The model under review builds one solid part; all positions refer to its coordinate system, in mm. A direction names the side the tool comes from. Coordinates: 2 decimals unless noted, no trailing zeros. Write each loop counter-clockwise with the first axis right and the second up, starting at its lowest first coordinate (ties: lowest second). Pieces come first, ordered by that corner, then holes. Notation, with made-up numbers: (66, -22.5) - (91, -22.5) arc R37 cw to (91, 16.5) - close; hole circle Ø9 at (-17.75, 47). An arc over 180 degrees is marked (long way). Use one line per item in the form item = value. Start each with the question number.
```python
from build123d import *

# Parameters (mm, degrees)
PAD004_DEPTH       = 23
PAD005_DEPTH       = 44
SKETCH007_W        = 43
SKETCH007_H        = 35
POCKET001_DEPTH    = 53
PAD006_DEPTH       = 25
SKETCH009_R        = 1.5
POCKET002_DEPTH    = 44.001
SKETCH012_R        = 3
POCKET004_DEPTH    = 10
POLARPATTERN_COUNT = 4
CHAMFER_SIZE       = 5
POCKET_DEPTH       = 5
PAD_DEPTH          = 44
SKETCH014_R        = 1.5
POCKET005_DEPTH    = 57.001
PAD007_DEPTH       = 15
SKETCH016_R        = 1.5
POCKET006_DEPTH    = 20
SKETCH017_R        = 1.5
POCKET007_DEPTH    = 20
SKETCH018_W        = 9
SKETCH018_H        = 10
POCKET008_DEPTH    = 15
POCKET009_DEPTH    = 15
SKETCH020_R        = 1.5
POCKET010_DEPTH    = 5


with BuildPart() as part:
    # Sketch005 → Pad004 (new body)
    with BuildSketch(Plane.XY):
        Polygon((32, -42), (32, 32), (-32, 32), (-32, -42), (-20, -42), (-20, 20), (20, 20), (20, -42), align=None)
    extrude(amount=-PAD004_DEPTH)

    # Sketch006 (on Face10 of Pad004) → Pad005 (join)
    with BuildSketch(Plane(origin=(0, 0, -23), x_dir=(1, 0, 0), z_dir=(0, 0, -1))):
        with BuildLine():
            Line((-25, 57), (-25, -1))
            Line((-25, -1), (25, -1))
            Line((25, -1), (25, 57))
            Line((25, 57), (12, 57))
            Line((12, 28.000302), (12, 57))
            ThreePointArc((-12, 27.999702), (0.0003, 16), (12, 28.000302))
            Line((-12, 27.999702), (-12, 57))
            Line((-12, 57), (-25, 57))
        make_face()
    extrude(amount=PAD005_DEPTH)

    # Sketch007 (on Face16 of Pad005) → Pocket001 (cut)
    with BuildSketch(Plane.XZ.offset(57)):
        with Locations((0, -45.217157)):
            Rectangle(SKETCH007_W, SKETCH007_H)
    extrude(amount=-POCKET001_DEPTH, mode=Mode.SUBTRACT)

    # Sketch008 (on Face9 of Pocket001) → Pad006 (join)
    with BuildSketch(Plane.XZ.offset(42)):
        Polygon((-32, -23), (-25, -23), (-25, -42.561909), align=None)
        Polygon((32, -23), (25, -23), (25, -42.561909), align=None)
    extrude(amount=-PAD006_DEPTH)

    # Sketch009 (on Face7 of Pad006) → Pocket002 (cut, through all)
    with BuildSketch(Plane.XY.offset(-23)):
        with Locations((-15.5, -12.5)):
            Circle(SKETCH009_R)
        with Locations((-15.5, -43.5)):
            Circle(SKETCH009_R)
        with Locations((15.5, -43.5)):
            Circle(SKETCH009_R)
        with Locations((15.5, -12.5)):
            Circle(SKETCH009_R)
    extrude(amount=-POCKET002_DEPTH, mode=Mode.SUBTRACT)

    # Sketch012 (on Face4 of Pocket002) → Pocket004 (cut)
    with BuildSketch(Plane.XY):
        with Locations((-25, 25)):
            Circle(SKETCH012_R)
    pocket004 = extrude(amount=-POCKET004_DEPTH, mode=Mode.SUBTRACT)

    # PolarPattern: Pocket004 ×4 about axis
    polarpattern_axis = Axis((0, 0, 0), (0, 0, 1))
    for i in range(1, POLARPATTERN_COUNT):
        add(pocket004.rotate(polarpattern_axis, i * 360 / POLARPATTERN_COUNT), mode=Mode.SUBTRACT)

    # Chamfer
    chamfer_edges = [part.edges().sort_by_distance(p)[0] for p in [
        (-32, 32, -11.5),
        (32, 32, -11.5),
        (-25, 1, -45),
        (25, 1, -45),
        (20, 20, -11.5),
        (-20, 20, -11.5),
    ]]
    chamfer(chamfer_edges, length=CHAMFER_SIZE)

    # Sketch013 (on Face37 of Chamfer) → Pocket (cut)
    with BuildSketch(Plane(origin=(0, 1, 0), x_dir=(-1, 0, 0), z_dir=(0, 1, 0))):
        with BuildLine():
            Line((-12, -62.717157), (12, -62.717157))
            Line((12, -62.717157), (12, -49.356773))
            ThreePointArc((12, -49.356773), (0, -37.356773), (-12, -49.356773))
            Line((-12, -49.356773), (-12, -62.717157))
        make_face()
    extrude(amount=-POCKET_DEPTH, mode=Mode.SUBTRACT)

    # Sketch (on Face5 of Pocket) → Pad (join)
    with BuildSketch(Plane(origin=(0, 0, -23), x_dir=(1, 0, 0), z_dir=(0, 0, -1))):
        Polygon((-32, 17), (-25, 17), (-25, 7), (-20, 2), (-20, -15), (-15, -20), (15, -20), (20, -15), (20, 2), (25, 7), (25, 17), (32, 17), (32, -27), (27, -32), (-27, -32), (-32, -27), align=None)
    extrude(amount=PAD_DEPTH)

    # Sketch014 (on Face13 of Pad) → Pocket005 (cut, through all)
    with BuildSketch(Plane(origin=(-25, 0, 0), x_dir=(0, -1, 0), z_dir=(-1, 0, 0))):
        with Locations((49.5, -33)):
            Circle(SKETCH014_R)
        with Locations((49.5, -56)):
            Circle(SKETCH014_R)
    extrude(amount=-POCKET005_DEPTH, mode=Mode.SUBTRACT)

    # Sketch015 (on Face26 of Pocket005) → Pad007 (join)
    with BuildSketch(Plane(origin=(-25, 0, 0), x_dir=(0, -1, 0), z_dir=(-1, 0, 0))):
        Polygon((22, -67), (42, -67), (42, -47), align=None)
    pad007 = extrude(amount=PAD007_DEPTH)

    # Sketch016 (on Face53 of Pad007) → Pocket006 (cut)
    with BuildSketch(Plane.XZ.offset(42)):
        with Locations((-32.5, -57)):
            Circle(SKETCH016_R)
    pocket006 = extrude(amount=-POCKET006_DEPTH, mode=Mode.SUBTRACT)

    # Sketch017 (on Face20 of Pocket006) → Pocket007 (cut)
    with BuildSketch(Plane(origin=(0, 0, -67), x_dir=(1, 0, 0), z_dir=(0, 0, -1))):
        with Locations((-32.5, 32)):
            Circle(SKETCH017_R)
    pocket007 = extrude(amount=-POCKET007_DEPTH, mode=Mode.SUBTRACT)

    # Sketch018 (on Face20 of Pocket007) → Pocket008 (cut)
    with BuildSketch(Plane(origin=(0, 0, -62), x_dir=(1, 0, 0), z_dir=(0, 0, -1))):
        with Locations((-32.5, 32)):
            Rectangle(SKETCH018_W, SKETCH018_H)
    pocket008 = extrude(amount=-POCKET008_DEPTH, mode=Mode.SUBTRACT)

    # Mirrored: Pad007, Pocket006, Pocket007, Pocket008 across YZ
    add(pad007.mirror(Plane.YZ))
    add(pocket006.mirror(Plane.YZ), mode=Mode.SUBTRACT)
    add(pocket007.mirror(Plane.YZ), mode=Mode.SUBTRACT)
    add(pocket008.mirror(Plane.YZ), mode=Mode.SUBTRACT)

    # Sketch019 (on Face5 of Mirrored) → Pocket009 (cut)
    with BuildSketch(Plane(origin=(0, 32, 0), x_dir=(-1, 0, 0), z_dir=(0, 1, 0))):
        with BuildLine():
            Line((-8, -63), (8, -63))
            Line((8, -63), (8, -50.411114))
            ThreePointArc((8, -50.411114), (0, -42.484996), (-8, -50.411114))
            Line((-8, -50.411114), (-8, -63))
        make_face()
    extrude(amount=-POCKET009_DEPTH, mode=Mode.SUBTRACT)

    # Sketch020 (on Face23 of Pocket009) → Pocket010 (cut)
    with BuildSketch(Plane.XY.offset(-63)):
        with Locations((0, 27.5)):
            Circle(SKETCH020_R)
    extrude(amount=-POCKET010_DEPTH, mode=Mode.SUBTRACT)


solid = part.part
```
1. For P1, Ø5, axis at y = 1.5, z = -36.5, coming from the +X side; P2, Ø4, axis at y = -45.5, z = -25.5, coming from the -X side; P3, Ø10, axis at x = 9.5, y = -29.5, coming from the +Z side, all flat-tipped, find the tip position at first contact; note any pin that passes through.
2. Take a section at D-D (x = 4.5). State the section outline as (y, z) points.
3. Take a section at C-C (z = -5). State the section outline as (x, y) points.
4. For L1, parallel to X at y = 5, z = -40; L2, parallel to Z at x = -3, y = -7.5; L3, parallel to Y at x = 15.5, z = -24.3, list the stretches that pass through material, from the lowest coordinate up.
5. For faces 4 (the flat face through (-30.7, -42, -57.1)), 5 (the flat face through (-34, -33, -62)), 6 (the flat face through (0, 20, -26)), 7 (the flat face through (-20, -8, -18)), 8 (the flat face through (-12, -42, -25)), list the 3-axis set-ups (+Z, -Z, +X, -X, +Y, -Y) from which the entire face can be reached by the end or side of a thin tool; tool diameter is ignored.
6. The part is to be moulded in two halves that separate along X. For faces 1 (the flat face through (30, 29, -33)), 2 (the flat face through (12, -42, -25)), 3 (the cylindrical face through (23.2, -48.3, -33.9)), say which applies: released by +X, released by -X, zero draft, split by the parting line, or undercut.
7. Take a section at B-B (z = -33). Count the separate pieces of the cut face and the enclosed holes in it, plus the area to 3 significant figures.
8. Take a section at A-A (y = -12.5). State the section outline as (x, z) points.
Returned:
q1.P1 = 32
q1.P2 = -25
q1.P3 = -23
q2.outline = (-16.88, -67) - (1, -67) - (1, -62.72) - (-16.88, -62.72) - close; (-16.88, -27.72) - (-4, -27.72) - (-4, -38.23) - (1, -38.23) - (1, -23) - (-16.88, -23) - close; (20, -67) - (32, -67) - (32, -63) - (20, -63) - close; (20, -43.87) - (32, -43.87) - (32, 0) - (20, 0) - close
q3.outline = (-32, -42) - (-20, -42) - (-20, 15) - (-15, 20) - (15, 20) - (20, 15) - (20, -42) - (32, -42) - (32, 27) - (27, 32) - (-27, 32) - (-32, 27) - close; hole circle Ø6 at (-25, -25); hole circle Ø6 at (-25, 25); hole circle Ø6 at (25, -25); hole circle Ø6 at (25, 25)
q4.L1 = -32 to -20, 20 to 32
q4.L2 = -67 to -62.72, -27.72 to -23
q4.L3 = -57 to -45, -42 to -14, -11 to 1, 19.5 to 32
q5.face_4 = +Z, -Z, -X, -Y
q5.face_5 = none
q5.face_6 = +Z, -Z
q5.face_7 = +Z
q5.face_8 = +Z, -Z, -Y
q6.face_1 = released by +X
q6.face_2 = undercut
q6.face_3 = zero draft
q7.separate_pieces = 3
q7.enclosed_holes = 1
q7.area = 2,250 mm²
q8.outline = (-32, -67) - (-17, -67) - (-17, -62.72) - (-21.5, -62.72) - (-21.5, -27.72) - (-17, -27.72) - (-17, -23) - (-20, -23) - (-20, 0) - (-32, 0) - close; (-14, -67) - (14, -67) - (14, -62.72) - (-14, -62.72) - close; (-14, -27.72) - (14, -27.72) - (14, -23) - (-14, -23) - close; (17, -67) - (32, -67) - (32, 0) - (20, 0) - (20, -23) - (17, -23) - (17, -27.72) - (21.5, -27.72) - (21.5, -62.72) - (17, -62.72) - close
